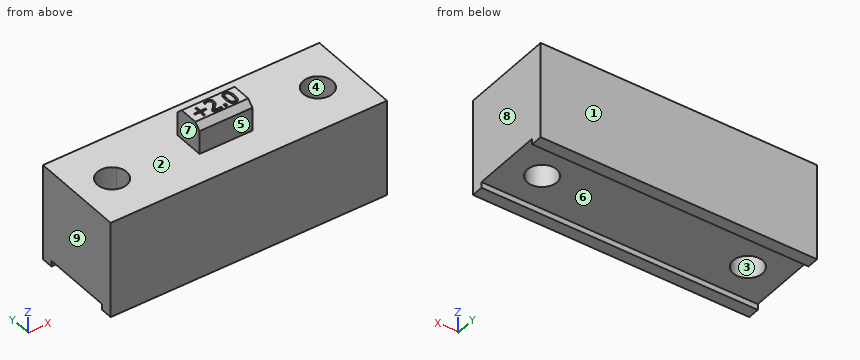
Autodesk Inventor part; units mm, degrees
ref_plane "YZ Plane" through (0, 0, 0) normal (1, 0, 0) x (0, 1, 0)
ref_plane "XZ Plane" through (0, 0, 0) normal (0, 1, 0) x (-1, 0, 0)
ref_plane "XY Plane" through (0, 0, 0) normal (0, 0, 1) x (1, 0, 0)
ref_plane "작업 평면1" through (23.5, -8, -2) normal (1, 0, 0) x (0, 0, -1)
sketch "스케치1" plane through (23.5, -8, -2) normal (1, 0, 0) x (0, 0, -1)
  line L0 (0, 16) -> (-8.15, 16)
  line L1 (-8.15, 16) -> (-8.15, 10.6)
  line L2 (-8.15, 10.6) -> (-12.15, 10.6)
  line L3 (-13.15, 9.6) -> (-12.15, 10.6)
  line L4 (-13.15, 9.6) -> (-13.15, 6.4)
  line L5 (-12.15, 5.4) -> (-13.15, 6.4)
  line L6 (-12.15, 5.4) -> (-8.15, 5.4)
  line L7 (-8.15, 5.4) -> (-8.15, 0)
  line L8 (-8.15, 0) -> (0, 0)
  line L9 (0, 16) -> (8.35, 16)
  line L10 (8.35, 16) -> (8.35, 15)
  line L11 (0, 0) -> (8.35, 0)
  line L12 (8.35, 0) -> (8.35, 1)
  line L13 (0, 16) -> (-8.15, 16)
  line L14 (-8.15, 10.6) -> (-12.15, 10.6)
  line L15 (-8.15, 10.6) -> (-12.15, 10.6)
  line L16 (-12.15, 10.6) -> (-13.15, 9.6)
  line L17 (-13.15, 6.4) -> (-12.15, 5.4)
  line L18 (7.35, 14) -> (8.35, 14)
  line L19 (8.35, 14) -> (8.35, 15)
  line L20 (7.35, 2) -> (8.35, 2)
  line L21 (8.35, 2) -> (8.35, 1)
  line L22 (7.35, 14) -> (7.35, 2)
  point P0 (-2, 8)
  point P1 (4.35, 10.6)
  point P2 (4.35, 5.4)
  dimension "d1" = 8.35
  dimension "d13" = 8.35
sketch "스케치2" plane through (-23.5, 8, 6.15) normal (0, 0, 1) x (1, 0, 0)
  arc A0 (7.9209, -9.6) -> (7.9209, -6.4) centre (6, -8) ccw
  line L0 (39.0791, -9.6) -> (7.9209, -9.6)
  circle A1 centre (6, -8) radius 2.5
  circle A2 centre (41, -8) radius 2.5
  circle A3 centre (41, -8) radius 2.5
  point P0 (23.5, -8)
  point P1 (7.9209, -6.4)
extrude "돌출1" add sketch "스케치1" against normal up to surface (47 mm away)
extrude "돌출2" cut sketch "스케치2" along normal mid plane 50
sketch "스케치3" plane through (-15.5791, 1.6, 11.15) normal (0, 0, 1) x (1, 0, 0)
  line L0 (15.5791, -14.4593) -> (15.5791, 15.5737)
  line L1 (-7.9209, 4.4) -> (-7.9209, -7.6)
  line L2 (-7.9209, 4.4) -> (11.0791, 4.4)
  line L3 (11.0791, 4.4) -> (11.0791, -7.6)
  line L4 (11.0791, -7.6) -> (-7.9209, -7.6)
  line L5 (-7.9209, -7.6) -> (-7.9209, 4.4)
  line L6 (39.0791, 4.4) -> (39.0791, -7.6)
  line L7 (39.0791, 4.4) -> (20.0791, 4.4)
  line L8 (20.0791, 4.4) -> (20.0791, -7.6)
  line L9 (20.0791, -7.6) -> (39.0791, -7.6)
  line L10 (39.0791, -7.6) -> (39.0791, 4.4)
  point P0 (15.5791, -1.6)
  dimension "d9" = 19
extrude "돌출3" cut sketch "스케치3" against normal up to surface (5 mm away)
sketch "스케치4" plane through (-4.5, 1.6, 11.15) normal (0, 0, 1) x (1, 0, 0)
  line L0 (0.6181, -0.2528) -> (7.2489, -0.2528) construction
  line L1 (7.2489, -0.2528) -> (7.2489, -2.6222) construction
  line L2 (7.2489, -2.6222) -> (0.6181, -2.6222) construction
  line L3 (0.6181, -2.6222) -> (0.6181, -0.2528) construction
  line L4 (2.8925, -1.8707) -> (2.0321, -1.8707)
  line L5 (2.0321, -1.8707) -> (2.0321, -2.7311)
  line L6 (2.0321, -2.7311) -> (1.7481, -2.7311)
  line L7 (1.7481, -2.7311) -> (1.7481, -1.8707)
  line L8 (1.7481, -1.8707) -> (0.8877, -1.8707)
  line L9 (0.8877, -1.8707) -> (0.8877, -1.5969)
  line L10 (0.8877, -1.5969) -> (1.7481, -1.5969)
  line L11 (1.7481, -1.5969) -> (1.7481, -0.7365)
  line L12 (1.7481, -0.7365) -> (2.0321, -0.7365)
  line L13 (2.0321, -0.7365) -> (2.0321, -1.5969)
  line L14 (2.0321, -1.5969) -> (2.8925, -1.5969)
  line L15 (2.8925, -1.5969) -> (2.8925, -1.8707)
  line L16 (4.9118, -2.8463) -> (3.3454, -2.8463)
  line L17 (3.3454, -2.8463) -> (3.3454, -2.4861)
  spline S0 degree 2 poles (3.3454, -2.4861) (3.5142, -2.3276) (3.8147, -2.0333) (3.9588, -1.8748) knots 0 0 0 1 2 2 2
  spline S1 degree 2 poles (3.9588, -1.8748) (4.249, -1.5558) (4.461, -1.1729) (4.461, -0.9691) knots 0 0 0 1 2 2 2
  spline S2 degree 2 poles (4.461, -0.9691) (4.461, -0.8621) (4.3951, -0.7015) (4.3354, -0.6501) knots 0 0 0 1 2 2 2
  spline S3 degree 2 poles (4.3354, -0.6501) (4.2757, -0.5986) (4.1193, -0.5472) (4.0246, -0.5472) knots 0 0 0 1 2 2 2
  spline S4 degree 2 poles (4.0246, -0.5472) (3.9341, -0.5472) (3.7488, -0.5925) (3.6644, -0.6274) knots 0 0 0 1 2 2 2
  spline S5 degree 2 poles (3.6644, -0.6274) (3.5924, -0.6563) (3.4586, -0.7386) (3.4174, -0.7674) knots 0 0 0 1 2 2 2
  line L18 (3.4174, -0.7674) -> (3.3989, -0.7674)
  line L19 (3.3989, -0.7674) -> (3.3989, -0.4051)
  spline S6 degree 2 poles (3.3989, -0.4051) (3.5039, -0.3537) (3.8805, -0.2528) (4.0493, -0.2528) knots 0 0 0 1 2 2 2
  spline S7 degree 2 poles (4.0493, -0.2528) (4.4054, -0.2528) (4.8068, -0.6295) (4.8068, -0.9506) knots 0 0 0 1 2 2 2
  spline S8 degree 2 poles (4.8068, -0.9506) (4.8068, -1.1009) (4.7368, -1.352) (4.6751, -1.459) knots 0 0 0 1 2 2 2
  spline S9 degree 2 poles (4.6751, -1.459) (4.6133, -1.5702) (4.4342, -1.7884) (4.3354, -1.8933) knots 0 0 0 1 2 2 2
  spline S10 degree 2 poles (4.3354, -1.8933) (4.1749, -2.0683) (3.7817, -2.4429) (3.6644, -2.552) knots 0 0 0 1 2 2 2
  line L20 (3.6644, -2.552) -> (4.9118, -2.552)
  line L21 (4.9118, -2.552) -> (4.9118, -2.8463)
  line L22 (5.7969, -2.8463) -> (5.3893, -2.8463)
  line L23 (5.3893, -2.8463) -> (5.3893, -2.3606)
  line L24 (5.3893, -2.3606) -> (5.7969, -2.3606)
  line L25 (5.7969, -2.3606) -> (5.7969, -2.8463)
  spline S11 degree 2 poles (7.8902, -1.5763) (7.8902, -2.2597) (7.4929, -2.8999) (7.0792, -2.8999) knots 0 0 0 1 2 2 2
  spline S12 degree 2 poles (7.0792, -2.8999) (6.6593, -2.8999) (6.2662, -2.2474) (6.2662, -1.5784) knots 0 0 0 1 2 2 2
  spline S13 degree 2 poles (6.2662, -1.5784) (6.2662, -0.8909) (6.6634, -0.2549) (7.0792, -0.2549) knots 0 0 0 1 2 2 2
  spline S14 degree 2 poles (7.0792, -0.2549) (7.4971, -0.2549) (7.8902, -0.9136) (7.8902, -1.5763) knots 0 0 0 1 2 2 2
  spline S15 degree 2 poles (7.4538, -2.3503) (7.5032, -2.2247) (7.5444, -1.8378) (7.5444, -1.5763) knots 0 0 0 1 2 2 2
  spline S16 degree 2 poles (7.5444, -1.5763) (7.5444, -1.3149) (7.5032, -0.93) (7.4518, -0.8003) knots 0 0 0 1 2 2 2
  spline S17 degree 2 poles (7.4518, -0.8003) (7.4003, -0.6707) (7.2212, -0.5369) (7.0792, -0.5369) knots 0 0 0 1 2 2 2
  spline S18 degree 2 poles (7.0792, -0.5369) (6.9372, -0.5369) (6.754, -0.6707) (6.7005, -0.8045) knots 0 0 0 1 2 2 2
  spline S19 degree 2 poles (6.7005, -0.8045) (6.649, -0.9341) (6.612, -1.3293) (6.612, -1.5784) knots 0 0 0 1 2 2 2
  spline S20 degree 2 poles (6.612, -1.5784) (6.612, -1.846) (6.6449, -2.2041) (6.6984, -2.3441) knots 0 0 0 1 2 2 2
  spline S21 degree 2 poles (6.6984, -2.3441) (6.7478, -2.4758) (6.931, -2.6179) (7.0792, -2.6179) knots 0 0 0 1 2 2 2
  spline S22 degree 2 poles (7.0792, -2.6179) (7.2192, -2.6179) (7.4024, -2.4841) (7.4538, -2.3503) knots 0 0 0 1 2 2 2
  point P0 (4.5, -1.6)
extrude "돌출4" cut sketch "스케치4" against normal blind 5
properties part number "Bearing Spacer_V2_2mm"
Geometry check sheet. Reference: the model listing, model coordinates, mm. Face numbers are marked on the shaded views. A direction names the side the tool comes from. Round coordinates to 2 decimals unless told otherwise and drop trailing zeros. Write each loop counter-clockwise with the first axis right and the second up, starting at its lowest first coordinate (ties: lowest second). Pieces come first, ordered by that corner, then holes. Notation, with made-up numbers: (63, 75.5) -> (107, 75.5) arc R16 ccw to (107, 94.5) -> close; hole circle Ø3 at (82.5, -30.75). An arc over 180 degrees is marked (long way). One line per item, written item: value. Start each with the question number.
(1) Cross-section at D-D, the plane y = 5.5. Record the cut outline in (x, z), and give its area (4 significant figures).
(2) Go/stop test with flat-tipped pins: pin 1 Ø2 at (x, z) = (-2, 9) entering from -Y; pin 2 Ø8 at (x, y) = (17.5, 0) entering from -Z; pin 3 Ø1 at (x, y) = (-2.5, 0) entering from +Z; pin 4 Ø2 at (x, y) = (-9, -4) entering from +Z. Record where each tip stops, or that it passes through.
(3) Access from +Z, -Z, +X, -X, +Y, -Y to the whole of each face (thin tool, end or side, straight path). Record for the marked faces 5, 6, 7, 8 and 9.
(4) Draft check along Y on the marked faces 1, 2, 3 and 4. Enter one of: +Y half, -Y half, draft (parallel to the pull), parting line (faces both ways), or undercut.
(5) Cross-section at C-C, the plane z = 0.5. Record the cut outline in (x, y), and give its area (3 significant figures).
(6) Cross-section at A-A, the plane x = -17.5. Record the cut outline in (y, z), and give its area (4 significant figures).
(7) Cross-section at B-B, the plane z = 9. Give the number of separate pieces and of enclosed holes in the cut face, and give its area (3 significant figures).
(8) Scan lines: line 1 (Y direction, x = -17.5, z = -1); line 2 (X direction, y = -1, z = 4.5); line 3 (Z direction, x = -10, y = 0.25). Record each from-to range of solid material in increasing order. Write a range as [from, to].
Answer:
1. outline: (-23.5, -9.35) -> (23.5, -9.35) -> (23.5, 6.15) -> (-23.5, 6.15) -> close
1. area: 728.5 mm²
2. pin 1: y = -2.6
2. pin 2: z = -9.35
2. pin 3: z = 11.15
2. pin 4: z = 6.15
3. face 5: +Z, +X, -X, -Y
3. face 6: -Z, +X, -X
3. face 7: +Z, -X, +Y, -Y
3. face 8: +Z, -Z, +X, +Y, -Y
3. face 9: +Z, -Z, -X, +Y, -Y
4. face 1: +Y half
4. face 2: draft
4. face 3: undercut
4. face 4: undercut
5. outline: (-23.5, -8) -> (23.5, -8) -> (23.5, 8) -> (-23.5, 8) -> close; hole circle Ø5 at (-17.5, 0); hole circle Ø5 at (17.5, 0)
5. area: 713 mm²
6. outline: (-8, -10.35) -> (-6, -10.35) -> (-6, -9.35) -> (-2.5, -9.35) -> (-2.5, 6.15) -> (-8, 6.15) -> close; (2.5, -9.35) -> (6, -9.35) -> (6, -10.35) -> (8, -10.35) -> (8, 6.15) -> (2.5, 6.15) -> close
6. area: 174.5 mm²
7. separate pieces: 2
7. enclosed holes: 4
7. area: 42.1 mm²
8. line 1: [-8, -2.5], [2.5, 8]
8. line 2: [-23.5, -19.79], [-15.21, 15.21], [19.79, 23.5]
8. line 3: [-9.35, 6.15]
